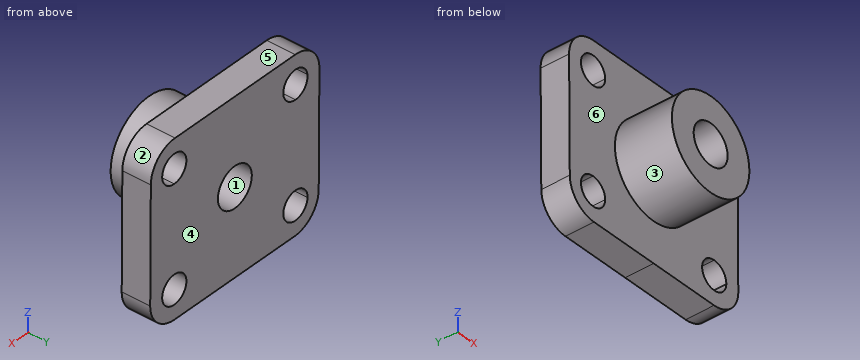
from build123d import *

# Parameters (mm, degrees)
F1_DEPTH = 10
F2_R     = 10
F3_R     = 16
F4_DEPTH = 20
F5_D     = 14
F5_DEPTH = 31
F5_TIP   = 4.2060243332


with BuildPart() as f1:
    # F0 (on Front) → F1 (new body)
    with BuildSketch(Plane.XZ):
        with BuildLine():
            ThreePointArc((-16, 0), (-11.313708499, 11.313708499), (0, 16))
            Line((0, 16), (0, 30))
            Line((0, 30), (-34.9625474322, 30))
            Line((-34.9625474322, 30), (-34.8962779592, 20.6108379355))
            Line((-34.8962779592, 20.6108379355), (-29.9625474322, 20.6108379355))
            ThreePointArc((-29.9625474322, 20.6108379355), (-24.6940074845, 24.9906280747), (-20, 20))
            ThreePointArc((-20, 20), (-21.4644660941, 16.4644660941), (-25, 15))
            Line((-25, 15), (-25, 0))
            Line((-25, 0), (-16, 0))
        make_face()
        with BuildLine():
            ThreePointArc((0, 16), (11.313708499, 11.313708499), (16, 0))
            Line((16, 0), (25, 0))
            Line((25, 0), (25, 15))
            ThreePointArc((25, 15), (21.4644660941, 23.5355339059), (30, 20))
            Line((30, 20), (34.6863753932, 20))
            Line((34.6863753932, 20), (34.6236340702, 30))
            Line((34.6236340702, 30), (0, 30))
            Line((0, 30), (0, 16))
        make_face()
        with BuildLine():
            Line((25, 0), (16, 0))
            ThreePointArc((16, 0), (11.313708499, -11.313708499), (0, -16))
            Line((0, -16), (0, -29.9935078941))
            Line((0, -29.9935078941), (35, -29.9869291484))
            Line((35, -29.9869291484), (34.9391447048, -20.2875329247))
            Line((34.9391447048, -20.2875329247), (29.9917256352, -20.2875329247))
            ThreePointArc((29.9917256352, -20.2875329247), (21.3642287872, -23.432370564), (25, -15))
            Line((25, -15), (25, 0))
        make_face()
        with BuildLine():
            Line((0, -29.9935078941), (0, -16))
            ThreePointArc((0, -16), (-11.313708499, -11.313708499), (-16, 0))
            Line((-16, 0), (-25, 0))
            Line((-25, 0), (-25, -15))
            ThreePointArc((-25, -15), (-21.4644660941, -16.4644660941), (-20, -20))
            ThreePointArc((-20, -20), (-24.9096942239, -24.9991844202), (-29.9967379467, -20.1805820915))
            Line((-29.9967379467, -20.1805820915), (-34.6083687837, -20.1805820915))
            Line((-34.6083687837, -20.1805820915), (-34.5390625298, -30))
            Line((-34.5390625298, -30), (0, -29.9935078941))
        make_face()
        with BuildLine():
            Line((-25, -15), (-25, 0))
            Line((-25, 0), (-25, 15))
            ThreePointArc((-25, 15), (-28.7452763368, 16.6874624287), (-29.9625474322, 20.6108379355))
            Line((-29.9625474322, 20.6108379355), (-34.8962779592, 20.6108379355))
            Line((-34.8962779592, 20.6108379355), (-34.6083687837, -20.1805820915))
            Line((-34.6083687837, -20.1805820915), (-29.9967379467, -20.1805820915))
            ThreePointArc((-29.9967379467, -20.1805820915), (-28.5988130305, -16.5288986227), (-25, -15))
        make_face()
        with BuildLine():
            Line((25, 15), (25, 0))
            Line((25, 0), (25, -15))
            ThreePointArc((25, -15), (28.5355339059, -16.4644660941), (30, -20))
            ThreePointArc((30, -20), (29.9979309807, -20.1438259781), (29.9917256352, -20.2875329247))
            Line((29.9917256352, -20.2875329247), (34.9391447048, -20.2875329247))
            Line((34.9391447048, -20.2875329247), (34.6863753932, 20))
            Line((34.6863753932, 20), (30, 20))
            ThreePointArc((30, 20), (28.5355339059, 16.4644660941), (25, 15))
        make_face()
        with BuildLine():
            ThreePointArc((-16, 0), (-11.313708499, -11.313708499), (0, -16))
            Line((0, -16), (0, 0))
            Line((0, 0), (-16, 0))
        make_face()
        with BuildLine():
            Line((0, 0), (0, 16))
            ThreePointArc((0, 16), (-11.313708499, 11.313708499), (-16, 0))
            Line((-16, 0), (0, 0))
        make_face()
        with BuildLine():
            Line((0, 0), (16, 0))
            ThreePointArc((16, 0), (11.313708499, 11.313708499), (0, 16))
            Line((0, 16), (0, 0))
        make_face()
        with BuildLine():
            ThreePointArc((0, -16), (11.313708499, -11.313708499), (16, 0))
            Line((16, 0), (0, 0))
            Line((0, 0), (0, -16))
        make_face()
    extrude(amount=F1_DEPTH)

    # F2
    f2_edges = [f1.edges().sort_by_distance(p)[0] for p in [
        (34.623634, -5, 30),
        (-34.962547, -5, 30),
        (35, -5, -29.986929),
        (-34.539063, -5, -30),
    ]]
    fillet(f2_edges, radius=F2_R)

    # F3 (on face) → F4 (join)
    with BuildSketch(Plane.XZ.offset(10)):
        Circle(F3_R)
    extrude(amount=F4_DEPTH)

    # F5
    with Locations(Plane(origin=(0, 0, 0), x_dir=(1, 0, 0), z_dir=(0, 1, 0))):
        with Locations((0, 0)):
            Hole(F5_D / 2, depth=F5_DEPTH)
            with Locations((0, 0, -(F5_DEPTH + F5_TIP / 2))):  # 118° drill point
                Cone(0, F5_D / 2, F5_TIP, mode=Mode.SUBTRACT)


solid = f1.part
Geometry check sheet. Reference: the model listing, model coordinates, mm. Face numbers are marked on the shaded views. A direction names the side the tool comes from. Round coordinates to 2 decimals unless told otherwise and drop trailing zeros. Order: outer loops, then holes, each group sorted by start corner. A loop starts at its lowest first (then second) coordinate and runs counter-clockwise, first axis right, second up. Notation, with made-up numbers: (64.25, -24.5) -> (77.25, -24.5) arc R34 ccw to (77.25, 10.5) -> close; hole circle Ø8 at (23.25, 86). An arc over 180 degrees is marked (long way). Use one line per item in the form item = value.
1. Set-up check for the marked faces 5 and 6: record each of +Z, -Z, +X, -X, +Y, -Y from which the full face is reachable in a straight line by a thin tool's end or side.
Working result:
face_5 = +Z, +X, -X, +Y, -Y
face_6 = -Y
2. Cross-section at D-D, the plane x = 13.5. Enter the section's corners in (y, z), plus the area to 3 significant figures.
Working result:
outline = (-30, -8.59) -> (-10, -8.59) -> (-10, -29.99) -> (0, -29.99) -> (0, 30) -> (-10, 30) -> (-10, 8.59) -> (-30, 8.59) -> close
area = 943 mm^2
3. Scan lines: line 1 along Z through (x, y) = (25, -4.5); line 2 along X through (y, z) = (-3, -20); line 3 along X through (y, z) = (-5, 20). Record each from-to range of solid material in increasing order. Write a range as from..to.
Working result:
line_1 = -29.99..-25, -15..15, 25..30
line_2 = -34.61..-30, -20..20, 30..34.94
line_3 = -34.89..-30, -20..20, 30..34.69
4. Cross-section at A-A, the plane z = 0. Enter the section's corners in (x, y), plus the area to 3 significant figures.
Working result:
outline = (-34.75, -10) -> (-16, -10) -> (-16, -30) -> (-7, -30) -> (-7, 0) -> (-34.75, 0) -> close; (7, -30) -> (16, -30) -> (16, -10) -> (34.81, -10) -> (34.81, 0) -> (7, 0) -> close
area = 916 mm^2
5. Cross-section at B-B, the plane y = -24. Enter the section's corners in (x, z), plus the area to 3 significant figures.
Working result:
outline = circle Ø32 at (0, 0); hole circle Ø14 at (0, 0)
area = 650 mm^2
6. Cross-section at C-C, the plane z = 11. Enter the section's corners in (x, y).
Working result:
outline = (-34.83, -10) -> (-11.62, -10) -> (-11.62, -30) -> (11.62, -30) -> (11.62, -10) -> (34.74, -10) -> (34.74, 0) -> (-34.83, 0) -> close
7. Mould release check, pull along X, two halves, no side actions. Record for the marked faces 1, 2, 3 and 4: pulls with the +X half, pulls with the -X half, needs draft (parallel to the pull), parting line crosses it, or undercut.
Working result:
face_1 = undercut
face_2 = pulls with the +X half
face_3 = parting line crosses it
face_4 = needs draft
8. Go/stop test with flat-tipped pins: pin 1 (3 mm diameter, centred on y = -23.5, z = -0.5, fed in from -X); pin 2 (8 mm diameter, centred on y = -23, z = 18.5, fed in from -X); pin 3 (10 mm diameter, centred on y = -9.5, z = -9, fed in from -X). Record where each tip stops, or that it passes through.
Working result:
pin_1 = -16
pin_2 = -6.76
pin_3 = -34.72
